Autodesk Fusion 360 part; units mm, degrees
sketch "Skizze1" plane through (0, 0, 0) normal (0, 1, 0) x (1, 0, 0)
  line L0 (1.75, 0) -> (22.5, 0)
  line L1 (0, -1.75) -> (0, -22.5)
  line L2 (-16.51, 36.83) -> (16.51, 36.83)
  line L3 (19.05, 34.29) -> (19.05, -34.29)
  line L4 (16.51, -36.83) -> (-16.51, -36.83)
  line L5 (-19.05, -34.29) -> (-19.05, 34.29)
  arc A0 (-16.51, 36.83) -> (-19.05, 34.29) centre (-16.51, 34.29) ccw
  arc A1 (19.05, 34.29) -> (16.51, 36.83) centre (16.51, 34.29) ccw
  arc A2 (16.51, -36.83) -> (19.05, -34.29) centre (16.51, -34.29) ccw
  arc A3 (-19.05, -34.29) -> (-16.51, -36.83) centre (-16.51, -34.29) ccw
  arc A4 (20.05, 34.29) -> (16.51, 37.83) centre (16.51, 34.29) ccw
  line L6 (-16.51, 37.83) -> (16.51, 37.83)
  arc A5 (-16.51, 37.83) -> (-20.05, 34.29) centre (-16.51, 34.29) ccw
  line L7 (-20.05, -34.29) -> (-20.05, 34.29)
  arc A6 (-20.05, -34.29) -> (-16.51, -37.83) centre (-16.51, -34.29) ccw
  line L8 (16.51, -37.83) -> (-16.51, -37.83)
  arc A7 (16.51, -37.83) -> (20.05, -34.29) centre (16.51, -34.29) ccw
  line L9 (20.05, 34.29) -> (20.05, -34.29)
  line L10 (-15.3, 31.75) -> (15.3, 31.75)
  line L11 (15.3, 31.75) -> (15.3, -4.85)
  line L12 (15.3, -4.85) -> (-15.3, -4.85)
  line L13 (-15.3, -4.85) -> (-15.3, 31.75)
  circle A8 centre (-16.51, 34.29) radius 1.2
  circle A9 centre (16.51, 34.29) radius 1.2
  circle A10 centre (-16.51, -34.29) radius 1.2
  circle A11 centre (16.51, -34.29) radius 1.2
  circle A12 centre (0, -14.83) radius 6.5
  line L14 (-6.35, -27.33) -> (6.35, -27.33)
  line L15 (6.35, -27.33) -> (6.35, -35.33)
  line L16 (6.35, -35.33) -> (-6.35, -35.33)
  line L17 (-6.35, -35.33) -> (-6.35, -27.33)
  point P0 (-19.05, 36.83)
  point P1 (19.05, 36.83)
  point P2 (-19.05, -36.83)
  dimension "d1" = 73.66
  dimension "d2" = 38.1
  dimension "d3" = 2.54
  dimension "d4" = -1
  dimension "d5" = 30.6
  dimension "d6" = 5.08
  dimension "d7" = 2.4
  dimension "d8" = 36.6
  dimension "d9" = 8
  dimension "d10" = 12.7
  dimension "d11" = 1.5
  dimension "d12" = 22
  dimension "d13" = 13
extrude "Extrusion1" add sketch "Skizze1" along normal blind 2 contours L2 L3 L4 L5 A0 A1 A2 A3 | A4 L6 A5 L7 A6 L8 A7 L9
sketch "Skizze2" plane through (0, 2, 0) normal (0, 1, 0) x (-1, 0, 0)
  circle A0 centre (16.51, -34.29) radius 1.2
  line L0 (-6.35, 35.33) -> (6.35, 35.33)
  line L1 (6.35, 35.33) -> (6.35, 27.33)
  line L2 (6.35, 27.33) -> (-6.35, 27.33)
  line L3 (-6.35, 27.33) -> (-6.35, 35.33)
  circle A1 centre (-16.51, 34.29) radius 1.2
  circle A2 centre (-16.51, -34.29) radius 1.2
  circle A3 centre (16.51, 34.29) radius 1.2
  line L4 (-15.3, 4.85) -> (15.3, 4.85)
  line L5 (15.3, 4.85) -> (15.3, -31.75)
  line L6 (15.3, -31.75) -> (-15.3, -31.75)
  line L7 (-15.3, -31.75) -> (-15.3, 4.85)
  circle A4 centre (0, 14.83) radius 6.5
  arc A5 (16.51, -37.83) -> (20.05, -34.29) centre (16.51, -34.29) ccw
  line L8 (20.05, -34.29) -> (20.05, 34.29)
  arc A6 (20.05, 34.29) -> (16.51, 37.83) centre (16.51, 34.29) ccw
  line L9 (16.51, 37.83) -> (-16.51, 37.83)
  arc A7 (-16.51, 37.83) -> (-20.05, 34.29) centre (-16.51, 34.29) ccw
  line L10 (-20.05, 34.29) -> (-20.05, -34.29)
  arc A8 (-20.05, -34.29) -> (-16.51, -37.83) centre (-16.51, -34.29) ccw
  line L11 (-16.51, -37.83) -> (16.51, -37.83)
  circle A9 centre (0, 14.83) radius 2.5
  dimension "d16" = 5
extrude "Extrusion2" add sketch "Skizze2" along normal blind 1 contours L0 L1 L2 L3 | A4 | A5 L8 A6 L9 A7 L10 A8 L11
fillet "Abrundung1" radius 1 8 edges at (0, 3, 37.83) (19.0132, 3, 36.7932) (20.05, 3, 0) (19.0132, 3, -36.7932) (0, 3, -37.83) (-19.0132, 3, -36.7932) (-20.05, 3, 0) (-19.0132, 3, 36.7932)
chamfer "Fase1" distance 1.2 angle 45 4 edges at (-15.3912, 3, 34.7239) (17.6288, 3, 34.7239) (-15.3912, 3, -33.8561) (17.6288, 3, -33.8561)
chamfer "Fase2" distance 1 angle 45 1 edges at (-6.0601, 2, 12.4795)
chamfer "Fase3" distance 0.5 angle 45 1 edges at (2.3308, 3, 15.734)
equation "d5 = 30.1 mm + 0.5 mm"
equation "d6 = ( 2.54 * 2 ) * 1 mm"
Here's how the part is built. I have some questions about the finished solid (model axes, mm). A direction names the side the tool comes from. Give positions to 0.01 mm unless a question says otherwise; leave off trailing zeros. Order: outer loops, then holes, each group sorted by start corner. A loop starts at its lowest first (then second) coordinate and runs counter-clockwise, first axis right, second up. Notation, with made-up numbers: (-28.5, 3.25) - (-8.5, 3.25) arc R17 cw to (-8.5, 11.25) - close; hole circle Ø4 at (36, -26). An arc over 180 degrees is marked (long way). Answer as a JSON object with one key per item and string values. Group by question number.
Item 1: Which directions (+Z, -Z, +X, -X, +Y, -Y) give clear straight access to the entire face, cutting with the end or side of a thin tool? Please do faces 1 (the flat face through (-2.4, 2, 13.7)), 2 (the flat face through (15.3, 1, -14)), 3 (the cylindrical face through (-18.985, 0.986, 36.821)).
Item 2: If we section it at C-C on z = 3: Please give me the cut outline in (x, y).
Item 3: If we section it at B-B on y = 0.5: Please give me the cut outline in (x, z), and give its area (3 significant figures).
Item 4: If we section it at A-A on z = 14.83: Please give me the cut outline in (x, y), and give its area (3 significant figures).
Item 5: Please list where these lines run through material, in increasing order: probe 1 along X at (y, z) = (0.75, 34.29); probe 2 along Z at (x, y) = (16.51, 0.75); probe 3 along Z at (x, y) = (0, 0.65).
Item 6: If we mould it in two halves opening along X, with no side actions, what happens to faces 4 (the cylindrical face through (-17.394, 0.887, 35.101)), 5 (the cylindrical face through (18.985, 0.986, -36.821)), 6 (the flat face through (0, 3, 9))? For each: pulls with the +X half, pulls with the -X half, needs draft (parallel to the pull), parting line crosses it, or undercut.
Result set:
{
 "1": {"face 1": "-Y", "face 2": "+Y, -Y", "face 3": "+Z, -X, +Y, -Y"},
 "2": {"outline": "(-20.05, 0) - (-15.3, 0) - (-15.3, 3) - (-19.05, 3) arc R1 ccw to (-20.05, 2) - close; (15.3, 0) - (20.05, 0) - (20.05, 2) arc R1 ccw to (19.05, 3) - (15.3, 3) - close"},
 "3": {"outline": "(-20.05, -34.29) arc R3.54 ccw to (-16.51, -37.83) - (16.51, -37.83) arc R3.54 ccw to (20.05, -34.29) - (20.05, 34.29) arc R3.54 ccw to (16.51, 37.83) - (-16.51, 37.83) arc R3.54 ccw to (-20.05, 34.29) - close; hole circle Ø2.4 at (-16.51, -34.29); hole circle Ø2.4 at (-16.51, 34.29); hole (-15.3, -31.75) - (15.3, -31.75) - (15.3, 4.85) - (-15.3, 4.85) - close; hole circle Ø13 at (0, 14.83); hole (-6.35, 27.33) - (6.35, 27.33) - (6.35, 35.33) - (-6.35, 35.33) - close; hole circle Ø2.4 at (16.51, -34.29); hole circle Ø2.4 at (16.51, 34.29)", "area": "1,650 mm²"},
 "4": {"outline": "(-20.05, 0) - (-6.5, 0) - (-6.5, 1) - (-5.5, 2) - (-2.5, 2) - (-2.5, 2.5) - (-3, 3) - (-19.05, 3) arc R1 ccw to (-20.05, 2) - close; (2.5, 2) - (5.5, 2) - (6.5, 1) - (6.5, 0) - (20.05, 0) - (20.05, 2) arc R1 ccw to (19.05, 3) - (3, 3) - (2.5, 2.5) - close", "area": "89.6 mm²"},
 "5": {"probe 1": "-20.05 to -17.71, -15.31 to -6.35, 6.35 to 15.31, 17.71 to 20.05", "probe 2": "-37.83 to -35.49, -33.09 to 33.09, 35.49 to 37.83", "probe 3": "-37.83 to -31.75, 4.85 to 8.33, 21.33 to 27.33, 35.33 to 37.83"},
 "6": {"face 4": "undercut", "face 5": "pulls with the +X half", "face 6": "needs draft"}
}
